Autodesk Inventor part; units mm, degrees
ref_plane "YZ Plane" through (0, 0, 0) normal (1, 0, 0) x (0, 1, 0)
ref_plane "XZ Plane" through (0, 0, 0) normal (0, 1, 0) x (-1, 0, 0)
ref_plane "XY Plane" through (0, 0, 0) normal (0, 0, 1) x (1, 0, 0)
sketch "Sketch1" plane through (0, 0, 0) normal (0, 1, 0) x (-1, 0, 0)
  circle A0 centre (0, 0) radius 16.7005
  circle A1 centre (0, 0) radius 20.32
  dimension "d1" = 33.401
  dimension "d2" = 40.64
extrude "Extrusion1" add sketch "Sketch1" along normal blind 38.1
sketch "Sketch2" plane through (0, 38.1, 0) normal (0, 1, 0) x (1, 0, 0)
  line L0 (0, 0) -> (0, 17.78) construction
  line L1 (0, 17.78) -> (-12.5588, 15.9743)
  circle A0 centre (0, 0) radius 20.32
  line L2 (0, 17.78) -> (12.5588, 15.9743)
  line L3 (-12.5588, 15.9743) -> (-12.5588, 21.0543)
  line L4 (-12.5588, 21.0543) -> (0, 21.0543)
  line L5 (12.5588, 15.9743) -> (12.5588, 21.0543)
  line L6 (12.5588, 21.0543) -> (0, 21.0543)
  dimension "d5" = 17.78
  dimension "d6" = 5.08
extrude "Extrusion2" add sketch "Sketch2" against normal blind 38.1 contours L1 A0 L2 | L3 L4 L6 L5 A0 picked at (-7.0969, 17.3675)
sketch "Sketch3" plane through (12.5588, 38.1, -21.0543) normal (0, 0, -1) x (-1, 0, 0)
  circle A0 centre (21.5758, -19.05) radius 1.2319
  line L0 (25.1176, -38.1) -> (0, -38.1)
  line L1 (25.1176, 0) -> (25.1176, -38.1)
  line L2 (12.5588, -38.1) -> (12.5588, 17.1945) construction
  circle A1 centre (3.5418, -19.05) radius 1.2319
  circle A2 centre (12.5588, -27.9654) radius 1.2319
  circle A3 centre (12.5588, -10.1346) radius 1.2319
  line L3 (25.1176, 0) -> (0, 0)
  dimension "d9" = 2.4638
  dimension "d10" = 19.05
  dimension "d12" = 18.034
  dimension "d13" = 2.4638
  dimension "d14" = 2.4638
  dimension "d16" = 10.1346
  dimension "d17" = 10.1346
extrude "Extrusion3" cut sketch "Sketch3" against normal blind 2.54
fillet "Fillet1" radius 1.27 4 edges at (0, 0, -21.0543) (-12.5588, 19.05, -21.0543) (12.5588, 19.05, -21.0543) (0, 38.1, -21.0543)
properties part number "ROV Motor couppling"
Check sheet for the modelled part. Datum: model origin and axes. Units: mm. A direction names the side the tool comes from. Give positions to 0.01 mm unless a question says otherwise; leave off trailing zeros. Write each loop counter-clockwise with the first axis right and the second up, starting at its lowest first coordinate (ties: lowest second). Pieces come first, ordered by that corner, then holes. Notation, with made-up numbers: (41, 36) -> (76, 36) arc R16 cw to (76, 57) -> close; hole circle Ø9 at (61, -36.75). An arc over 180 degrees is marked (long way). Write item = value, one per line.
Item 1: Scan lines: probe 1 along Y at (x, z) = (0, -19.4); probe 2 along Y at (x, z) = (-1, -19); probe 3 along Z at (x, y) = (-1, 13.5). Record each from-to range of solid material in increasing order. Write a range as from..to.
Output:
probe_1 = 0..8.9, 11.37..26.73, 29.2..38.1
probe_2 = 0..9.42, 10.85..27.25, 28.68..38.1
probe_3 = -21.05..-16.67, 16.67..20.3
Item 2: Sectioned sample at D-D on z = 8.5. Record the boundary of the cut face in (x, y), and give its area (3 significant figures).
Output:
outline = (-18.46, 0) -> (-14.38, 0) -> (-14.38, 38.1) -> (-18.46, 38.1) -> close; (14.38, 0) -> (18.46, 0) -> (18.46, 38.1) -> (14.38, 38.1) -> close
area = 311 mm^2
Item 3: Tool access check on faces 4 (the cylindrical face through (-9.68, 20.09, -19.8)), 5 (the flat face through (-12.559, 19, -18)), 6 (the flat face through (11, 38.1, -13)). Record the directions out of +Z, -Z, +X, -X, +Y, -Y that give a thin tool (end or side, any length) a straight path to the whole face; none if there is none.
Output:
face_4 = -Z
face_5 = -Z, -X, +Y, -Y
face_6 = +Z, -Z, +X, -X, +Y
Item 4: Gauge pin test, flat ends, axial feed: pin 1 (2 mm diameter, centred on x = 0, y = 10.13, fed in from -Z); pin 2 (4 mm diameter, centred on x = 11.5, y = 12, fed in from +Z); pin 3 (4 mm diameter, centred on y = 27, z = -17.5, fed in from -X). Record the tip position at first contact, or that the pin passes through.
Output:
pin_1 = -18.51
pin_2 = 17.96
pin_3 = -13.14
Item 5: Sectioned sample at C-C on y = 34.5. Record the boundary of the cut face in (x, z), and give its area (3 significant figures).
Output:
outline = (-12.56, -19.78) arc R1.27 ccw to (-11.29, -21.05) -> (11.29, -21.05) arc R1.27 ccw to (12.56, -19.78) -> (12.56, -15.97) arc R20.32 ccw (long way) to (-12.56, -15.97) -> close; hole circle Ø33.4 at (0, 0)
area = 473 mm^2
Item 6: Sectioned sample at B-B on z = 0. Record the boundary of the cut face in (x, y), and give its area (3 significant figures).
Output:
outline = (-20.32, 0) -> (-16.7, 0) -> (-16.7, 38.1) -> (-20.32, 38.1) -> close; (16.7, 0) -> (20.32, 0) -> (20.32, 38.1) -> (16.7, 38.1) -> close
area = 276 mm^2
Item 7: Release check for a two-part mould opening along X. For faces 1 (the cylindrical face through (-0.18, 37.74, -20.67)), 2 (the flat face through (12.559, 19, -18)), 3 (the flat face through (-9, 19, -18.514)) record: +X half, -X half, draft (parallel to the pull), parting line (faces both ways), or undercut.
Output:
face_1 = draft
face_2 = +X half
face_3 = undercut
Item 8: Sectioned sample at A-A on x = 0. Record the boundary of the cut face in (y, z), and give its area (3 significant figures).
Output:
outline = (0, -19.78) arc R1.27 ccw to (1.27, -21.05) -> (8.9, -21.05) -> (8.9, -18.51) -> (11.37, -18.51) -> (11.37, -21.05) -> (26.73, -21.05) -> (26.73, -18.51) -> (29.2, -18.51) -> (29.2, -21.05) -> (36.83, -21.05) arc R1.27 ccw to (38.1, -19.78) -> (38.1, -16.7) -> (0, -16.7) -> close; (0, 16.7) -> (38.1, 16.7) -> (38.1, 20.32) -> (0, 20.32) -> close
area = 291 mm^2
